Verification items for the finished model (mm, model axes). A direction names the side the tool comes from. Coordinates: 2 decimals unless noted, no trailing zeros. Order: outer loops, then holes, each group sorted by start corner. A loop starts at its lowest first (then second) coordinate and runs counter-clockwise, first axis right, second up. Notation, with made-up numbers: M 73,30.25 L 77,30.25 A10 ccw 77,36.25 Z; hole C -3.75,80 d8. An arc over 180 degrees is marked long. Return JSON: item names as keys, results as strings. Group by question number.
Q1. Section check C-C, the plane x = 13.5. Enter the section's corners in (y, z).
Q2. Thickness scan on probe 1 along X at (y, z) = (2.5, -95); probe 2 along Z at (x, y) = (31.5, 8.25); probe 3 along Z at (x, y) = (85, 2.8). Record the ranges inside material, lowest first.
Q3. Section check A-A, the plane x = 85. Enter the section's corners in (y, z), then the cut area to 3 significant figures.
Q4. Go/stop test with flat-tipped pins: pin 1 Ø5 at (y, z) = (13, -49.5) entering from +X; pin 2 Ø8 at (x, y) = (34, 20.5) entering from -Z; pin 3 Ø6 at (x, y) = (33.5, 16.5) entering from +Z. Record where each tip stops, or that it passes through.
Q5. Mould release check, pull along Z, two halves, no side actions. Record for faces 4 (the face through (43, 0, -47)), 5 (the face through (42, 7, -15.5)), 6 (the face through (42, 7, -11.5)): pulls with the +Z half, pulls with the -Z half, needs draft (parallel to the pull), parting line crosses it, or undercut.
Q6. Access from +Z, -Z, +X, -X, +Y, -Y to the whole of each face (thin tool, end or side, straight path). Record for faces 1 (the face through (21, 3, -42.5)), 2 (the face through (17, 6, -52.5)), 3 (the face through (42, 2, 4)).
Q7. Section check B-B, the plane z = 0. Enter the section's corners in (x, y).
Q8. Section check D-D, the plane z = -69. Enter the section's corners in (x, y).
Autodesk Inventor part; units mm, degrees
ref_plane "YZ Plane" through (0, 0, 0) normal (1, 0, 0) x (0, 1, 0)
ref_plane "XZ Plane" through (0, 0, 0) normal (0, 1, 0) x (-1, 0, 0)
ref_plane "XY Plane" through (0, 0, 0) normal (0, 0, 1) x (1, 0, 0)
sketch "Náčrt1" plane through (0, 0, 0) normal (0, 1, 0) x (-1, 0, 0)
  line L0 (0, 0) -> (-85, 0)
  line L1 (-85, 0) -> (-85, -95)
  line L2 (-85, -95) -> (0, -95)
  line L3 (0, -95) -> (0, 0)
  line L4 (4, 4) -> (-89, 4)
  line L5 (-89, 4) -> (-89, -99)
  line L6 (-89, -99) -> (4, -99)
  line L7 (4, -99) -> (4, 4)
  circle A0 centre (0, 0) radius 2
  circle A1 centre (0, -95) radius 2
  circle A2 centre (-85, -95) radius 2
  circle A3 centre (-85, 0) radius 2
  dimension "d0" = 4
  dimension "d1" = 4
  dimension "d2" = 4
  dimension "d3" = 4
  dimension "d4" = 85
  dimension "d5" = 95
  dimension "d6" = 4
  dimension "d7" = 4
  dimension "d8" = 4
  dimension "d9" = 4
  dimension "d10" = 4
  dimension "d11" = 4
extrude "Vysunutí1" add sketch "Náčrt1" along normal blind 5 contours L0 A0 L3 A1 L2 A2 L1 A3 | L7 L6 L5 L4
extrude "Vysunutí2" cut sketch "Náčrt1" along normal blind 5 contours A3 L1 L0 | L0 L1 A3 | A0 L3 L0 | L0 L3 A0 | A2 L2 L1 | L1 L2 A2 | A1 L2 L3 | L3 L2 A1
fillet "Zaoblení1" radius 2 4 edges at (89, 2.5, 4) (-4, 2.5, 4) (89, 2.5, -99) (-4, 2.5, -99)
sketch "Náčrt2" plane through (0, 5, 0) normal (0, 1, 0) x (1, 0, 0)
  point P0 (0, 0)
ref_plane "Pracovní rovina1" through (87, 0, -47.5) normal (0, 0, -1) x (-1, 0, 0)
sketch "Náčrt3" plane through (87, 0, -47.5) normal (0, 0, -1) x (-1, 0, 0)
  line L0 (89, 5) -> (0, 5)
  line L1 (24.5, 5) -> (64.5, 5)
  line L2 (64.5, 5) -> (44.5, 25)
  line L3 (44.5, 25) -> (24.5, 5)
  line L4 (24.5, 5) -> (64.5, 5)
  line L5 (91, 0) -> (91, 5)
  point P0 (87, 0)
  dimension "d22" = 90
  dimension "d26" = 45
  dimension "d27" = 20
  dimension "d28" = 46.5
extrude "Vysunutí3" add sketch "Náčrt3" along normal mid plane 30
fillet "Zaoblení2" radius 2 1 edges at (42.5, 25, -47.5)
sketch "Náčrt4" plane through (0, 5, 0) normal (0, 1, 0) x (1, 0, 0)
  line L0 (11.5, 15.5) -> (73.5, 15.5)
  line L1 (73.5, 15.5) -> (73.5, 81.5)
  line L2 (73.5, 81.5) -> (11.5, 81.5)
  line L3 (11.5, 81.5) -> (11.5, 15.5)
  line L4 (7.5, 11.5) -> (77.5, 11.5)
  line L5 (77.5, 11.5) -> (77.5, 85.5)
  line L6 (77.5, 85.5) -> (7.5, 85.5)
  line L7 (7.5, 85.5) -> (7.5, 11.5)
  line L8 (-22.6, 47.5) -> (107.6, 47.5)
  line L9 (-4, 97) -> (-4, -2)
  line L10 (89, -2) -> (89, 97)
  point P0 (0, 0)
  dimension "d32" = 62
  dimension "d33" = 66
  dimension "d34" = 4
  dimension "d35" = 4
  dimension "d36" = 4
  dimension "d37" = 4
  dimension "d38" = 34
  dimension "d39" = 11.5
  dimension "d40" = 11.5
extrude "Vysunutí4" add sketch "Náčrt4" along normal blind 4 contours L0 L1 L8 L5 L4 L7 L3 | L8 L7 L6 L5 L1 L2 L3
sketch "Náčrt5" plane through (0, 5, 0) normal (0, 1, 0) x (1, 0, 0)
  line L0 (67, 42.5) -> (70, 42.5)
  line L1 (70, 42.5) -> (70, 52.5)
  line L2 (70, 52.5) -> (67, 52.5)
  line L3 (67, 52.5) -> (67, 42.5)
  line L4 (73.5, 81.5) -> (73.5, 15.5)
  line L5 (-22.6, 47.5) -> (107.6, 47.5)
  line L6 (15, 42.5) -> (18, 42.5)
  line L7 (18, 42.5) -> (18, 52.5)
  line L8 (18, 52.5) -> (15, 52.5)
  line L9 (15, 52.5) -> (15, 42.5)
  line L10 (11.5, 15.5) -> (11.5, 81.5)
  point P0 (0, 0)
  dimension "d43" = 3.5
  dimension "d44" = 3
  dimension "d45" = 10
  dimension "d46" = 5
  dimension "d47" = 5
  dimension "d48" = 10
  dimension "d49" = 3
  dimension "d50" = 3.5
extrude "Vysunutí5" add sketch "Náčrt5" along normal blind 3
sketch "Náčrt6" plane through (62.5, 5, -62.5) normal (0.7071, 0.7071, 0) x (-0.7071, 0.7071, 0)
  circle A0 centre (23.2843, 17) radius 1
  circle A1 centre (23.2843, 7.5) radius 1
  line L0 (26.2843, 0) -> (0, 0)
  line L1 (26.2843, 30) -> (26.2843, 0)
  point P0 (40.6586, 62.5)
  dimension "d53" = 9.5
  dimension "d54" = 2
  dimension "d55" = 2
  dimension "d56" = 7.5
  dimension "d57" = 3
  dimension "d58" = 3
sketch "Náčrt7" plane through (22.5, 5, -62.5) normal (-0.7071, 0.7071, 0) x (-0.7071, -0.7071, 0)
  circle A0 centre (-23.2843, 13) radius 1
  circle A1 centre (-23.2843, 22.5) radius 1
  line L0 (-26.2843, 0) -> (-26.2843, 30)
  line L1 (-26.2843, 30) -> (0, 30)
  point P0 (19.4454, 62.5)
  dimension "d59" = 2
  dimension "d60" = 2
  dimension "d61" = 9.5
  dimension "d62" = 3
  dimension "d63" = 3
  dimension "d64" = 7.5
extrude "Vysunutí6" cut sketch "Náčrt6" against normal blind 5
extrude "Vysunutí7" cut sketch "Náčrt7" against normal blind 5
sketch "Náčrt8" plane through (0, 5, 0) normal (0, 1, 0) x (1, 0, 0)
  line L0 (62.5, 62.5) -> (62.5, 32.5)
  line L1 (62.5, 42.5) -> (65.5, 42.5)
  line L2 (65.5, 42.5) -> (65.5, 52.5)
  line L3 (65.5, 52.5) -> (62.5, 52.5)
  line L4 (62.5, 52.5) -> (62.5, 42.5)
  line L5 (70, 52.5) -> (67, 52.5)
  line L6 (67, 42.5) -> (70, 42.5)
  line L7 (-22.6, 47.5) -> (107.6, 47.5)
  line L8 (22.5, 32.5) -> (22.5, 62.5)
  line L9 (22.5, 42.5) -> (19.5, 42.5)
  line L10 (19.5, 42.5) -> (19.5, 52.5)
  line L11 (19.5, 52.5) -> (22.5, 52.5)
  line L12 (22.5, 52.5) -> (22.5, 42.5)
  line L13 (15, 42.5) -> (18, 42.5)
  point P0 (0, 0)
  dimension "d69" = 10
  dimension "d70" = 5
  dimension "d73" = 5
  dimension "d74" = 10
extrude "Vysunutí8" cut sketch "Náčrt8" against normal blind 5 contours L3 L2 L7 L0 | L7 L2 L1 L0
extrude "Vysunutí9" cut sketch "Náčrt8" against normal blind 5 contours L8 L9 L10 L7 | L7 L10 L11 L8
sketch "Náčrt9" plane through (87, 0, -62.5) normal (0, 0, -1) x (-1, 0, 0)
  circle A0 centre (44.6005, 12.1716) radius 6
  arc A1 (45.9142, 23.5858) -> (43.0858, 23.5858) centre (44.5, 22.1716) ccw
  line L0 (64.5, 5) -> (45.9142, 23.5858)
  line L1 (43.0858, 23.5858) -> (24.5, 5)
  point P0 (87, 0)
  dimension "d77" = 12
  dimension "d78" = 10
  dimension "d79" = 9
  dimension "d80" = 9.1421
extrude "Vysunutí10" cut sketch "Náčrt9" against normal blind 30
equation "\"d1\" = d0"
equation "\"d2\" = d0"
equation "\"d3\" = d0"
equation "\"d9\" = d7"
equation "\"d10\" = d7"
equation "\"d11\" = d7"
equation "\"d35\" = d34"
equation "\"d36\" = d34"
equation "\"d37\" = d34"
equation "\"d55\" = d54"
equation "\"d58\" = d57"
equation "\"d60\" = d59"
equation "\"d63\" = d62"
properties part number "Senzor-vikos"
Numbers:
{
 "1": {"outline": "M 0,-99 L 5,-99 L 5,-85.5 L 9,-85.5 L 9,-81.5 L 5,-81.5 L 5,-15.5 L 9,-15.5 L 9,-11.5 L 5,-11.5 L 5,4 L 0,4 Z"},
 "2": {"probe 1": "x = -4 to -2, 2 to 83, 87 to 89", "probe 2": "z = -85.5 to -81.5, -62.5 to -32.5, -15.5 to -11.5", "probe 3": "z = -99 to -97, -93 to -2, 2 to 4"},
 "3": {"outline": "M 0,-99 L 5,-99 L 5,-97 L 0,-97 Z; M 0,-93 L 5,-93 L 5,-2 L 0,-2 Z; M 0,2 L 5,2 L 5,4 L 0,4 Z", "area": "475 mm2"},
 "4": {"pin 1": "stops at x = 57", "pin 2": "stops at z = -62.5", "pin 3": "stops at z = -32.5"},
 "5": {"face 4": "needs draft", "face 5": "undercut", "face 6": "pulls with the +Z half"},
 "6": {"face 1": "+Y, -Y", "face 2": "+Y", "face 3": "+Z, +X, -X, +Y, -Y"},
 "7": {"outline": "M -4,0 L -2,0 L -2,5 L -4,5 Z; M 2,0 L 83,0 L 83,5 L 2,5 Z; M 87,0 L 89,0 L 89,5 L 87,5 Z"},
 "8": {"outline": "M -4,0 L 89,0 L 89,5 L 77.5,5 L 77.5,9 L 73.5,9 L 73.5,5 L 11.5,5 L 11.5,9 L 7.5,9 L 7.5,5 L -4,5 Z"}
}
